Can you work these out from the model? Positions are in its coordinate system, mm. A direction names the side the tool comes from. Coordinates: 2 decimals unless noted, no trailing zeros. Loops run counter-clockwise (first coordinate to the right, second up) from the corner with the lowest first, then second, coordinate; pieces in that order, holes last. Notation, with made-up numbers: M -36,-8 L -17,-8 A26 cw -17,7 Z; hole C -24,-0.5 d2. An arc over 180 degrees is marked long. Answer as a JSON object with one key per item and string values. Group by question number.
Item 1: Suppose I cut it at B-B (x = 0). Write out the boundary of the cut face in (y, z).
Item 2: I'm going to push flat-ended pins straight in: pin 1 Ø4 at (x, y) = (-24.5, -122.5) entering from -Z; pin 2 Ø6 at (x, z) = (15, 181.5) entering from -Y; pin 3 Ø4 at (x, z) = (18, 160) entering from +Y; pin 4 Ø9 at (x, y) = (-21.15, -90) entering from +Z. Where does each tip first touch, or does it pass through?
Item 3: Suppose I cut it at C-C (z = 225). Write out the boundary of the cut face in (x, y), then the cut area to 3 significant figures.
Item 4: Suppose I cut it at A-A (y = 82). Write out the boundary of the cut face in (x, z).
Item 5: Suppose I cut it at D-D (y = -151). Write out the boundary of the cut face in (x, z), then the cut area to 3 significant figures.
Item 6: If I drill on line 1 (Y direction, x = -21, z = 257); line 2 (Y direction, x = -28, z = 103); line 3 (Z direction, x = -21, y = -4), over which ranges is the centre line in solid material (lowest first)?
Item 7: We'd pull the mould along X, two halves only. Please class faces 6 (the flat face through (1, -195, 258)), 7 (the flat face through (-40, -6, 161)), 8 (the cylindrical face through (-19, -36.627, 258.256)): +X half, -X half, draft (parallel to the pull), parting line (faces both ways), or undercut.
Item 8: Which directions (+Z, -Z, +X, -X, +Y, -Y) give clear straight access to the entire face, cutting with the end or side of a thin tool? Please do faces 1 (the flat face through (9, 0, 184)), 2 (the flat face through (9, -8, 129)), 3 (the flat face through (4, 20, 146)), 4 (the flat face through (-4, 20, 146)), 5 (the flat face through (1, 0, 49)).
```python
from build123d import *

# Parameters (mm, degrees)
F1_DEPTH = 40
F2_DEPTH = 4
F3_R     = 4
F4_DEPTH = 262.201
F5_R     = 6
F6_DEPTH = 124.001
F7_R     = 6
F8_DEPTH = 108.001


# Not quite as in the source:
# - a pattern or mirror of a feature is missing from the dataset's text; its kind, count and spacing are read off the source's solid


with BuildPart() as f1:
    # F0 (on Right) → F1 (new body, symmetric)
    with BuildSketch(Plane.YZ):
        Polygon((0, 262.2), (-195, 262.2), (-195, 254.2), (-175, 254.2), (-8, 254.2), (-8, 20), (-8, 0), (0, 0), (0, 100), (0, 108), (0, 242.2), align=None)
        Polygon((74.1, 108), (0, 108), (0, 100), (116, 100), (116, 108), align=None)
    extrude(amount=F1_DEPTH, both=True)

    # F0 (on Right) → F2 (join, symmetric)
    with BuildSketch(Plane.YZ):
        Polygon((-8, 254.2), (-175, 254.2), (-8, 20), align=None)
        Polygon((74.1, 108), (0, 242.2), (0, 108), align=None)
    extrude(amount=F2_DEPTH, both=True)

    # F3 (on face) → F4 (cut, through all)
    with BuildSketch(Plane.XY.offset(262.2)):
        with Locations((-21.15, -40)):
            Circle(F3_R)
        with Locations((-21.15, -90)):
            Circle(F3_R)
        with Locations((-21.15, -165)):
            Circle(F3_R)
    f4 = extrude(amount=-F4_DEPTH, mode=Mode.SUBTRACT)

    # F4_copies: F4 across plane
    add(f4.mirror(Plane(origin=(0, 0, 0), x_dir=(0, 0, 1), z_dir=(1, 0, 0))), mode=Mode.SUBTRACT)

    # F5 (on face) → F6 (cut, through all)
    with BuildSketch(Plane.XZ.offset(8)):
        with Locations((-21.15, 25)):
            Circle(F5_R)
    f6 = extrude(amount=-F6_DEPTH, mode=Mode.SUBTRACT)

    # F6_copies: F6 across plane
    add(f6.mirror(Plane(origin=(0, 0, 0), x_dir=(0, 0, 1), z_dir=(1, 0, 0))), mode=Mode.SUBTRACT)

    # F7 (on face) → F8 (cut, through all)
    with BuildSketch(Plane.XY.offset(108)):
        with Locations((-28, 104)):
            Circle(F7_R)
        with Locations((0, 82)):
            Circle(F7_R)
        with Locations((28, 104)):
            Circle(F7_R)
    extrude(amount=-F8_DEPTH, mode=Mode.SUBTRACT)


solid = f1.part
```
From the geometry:
{
 "1": {"outline": "M -195,254.2 L -175,254.2 L -8,20 L -8,0 L 0,0 L 0,100 L 76,100 L 76,108 L 74.1,108 L 0,242.2 L 0,262.2 L -195,262.2 Z; M 88,100 L 116,100 L 116,108 L 88,108 Z"},
 "2": {"pin 1": "z = 254.2", "pin 2": "y = -8", "pin 3": "y = 0", "pin 4": "z = 262.2"},
 "3": {"outline": "M -40,-8 L -4,-8 L -4,-154.18 L 4,-154.18 L 4,-8 L 40,-8 L 40,0 L 4,0 L 4,9.5 L -4,9.5 L -4,0 L -40,0 Z", "area": "1,890 mm2"},
 "4": {"outline": "M -40,100 L -6,100 L -6,108 L -40,108 Z; M 6,100 L 40,100 L 40,108 L 6,108 Z"},
 "5": {"outline": "M -40,254.2 L -4,254.2 L -4,220.54 L 4,220.54 L 4,254.2 L 40,254.2 L 40,262.2 L -40,262.2 Z", "area": "909 mm2"},
 "6": {"line 1": "-195 to -169, -161 to -94, -86 to -44, -36 to 0", "line 2": "-8 to 98, 110 to 116", "line 3": "0 to 19, 31 to 262.2"},
 "7": {"face 6": "draft", "face 7": "-X half", "face 8": "undercut"},
 "8": {"face 1": "+Z, +Y", "face 2": "-Z, -Y", "face 3": "+Z, +X, +Y", "face 4": "+Z, -X, +Y", "face 5": "-Z, +X, -X, +Y"}
}
